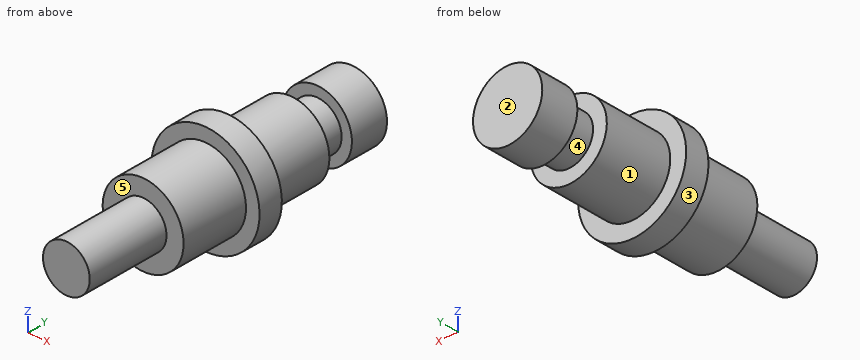
```python
from build123d import *

# Parameters (mm, degrees)
SKETCH1_R           = 4.77
BOSS_EXTRUDE1_DEPTH = 2.18
SKETCH2_R           = 3.575
BOSS_EXTRUDE2_DEPTH = 6.1
SKETCH3_R           = 2.065
BOSS_EXTRUDE3_DEPTH = 7.5
SKETCH4_R           = 3.365
BOSS_EXTRUDE4_DEPTH = 6.2
SKETCH5_R           = 2.15
BOSS_EXTRUDE5_DEPTH = 2.54
SKETCH6_R           = 3.06
BOSS_EXTRUDE6_DEPTH = 3.43


with BuildPart() as part:
    # Sketch1 → Boss-Extrude1 (new body)
    with BuildSketch(Plane(origin=(0, 0, 0), x_dir=(1, 0, 0), z_dir=(0, 1, 0))):
        with Locations(Location((0, 0, 0), (0, 0, 270))):
            Circle(SKETCH1_R)
    extrude(amount=BOSS_EXTRUDE1_DEPTH)

    # Sketch2 → Boss-Extrude2 (add)
    with BuildSketch(Plane.XZ):
        with Locations(Location((0, 0, 0), (0, 0, 90))):
            Circle(SKETCH2_R)
    extrude(amount=BOSS_EXTRUDE2_DEPTH)

    # Sketch3 → Boss-Extrude3 (add)
    with BuildSketch(Plane.XZ.offset(6.1)):
        with Locations(Location((0, 0, 0), (0, 0, 270))):
            Circle(SKETCH3_R)
    extrude(amount=BOSS_EXTRUDE3_DEPTH)

    # Sketch4 → Boss-Extrude4 (add)
    with BuildSketch(Plane(origin=(0, 2.18, 0), x_dir=(1, 0, 0), z_dir=(0, 1, 0))):
        with Locations(Location((0, 0, 0), (0, 0, 90))):
            Circle(SKETCH4_R)
    extrude(amount=BOSS_EXTRUDE4_DEPTH)

    # Sketch5 → Boss-Extrude5 (add)
    with BuildSketch(Plane(origin=(0, 8.38, 0), x_dir=(1, 0, 0), z_dir=(0, 1, 0))):
        with Locations(Location((0, 0, 0), (0, 0, 270))):
            Circle(SKETCH5_R)
    extrude(amount=BOSS_EXTRUDE5_DEPTH)

    # Sketch6 → Boss-Extrude6 (add)
    with BuildSketch(Plane(origin=(0, 10.92, 0), x_dir=(1, 0, 0), z_dir=(0, 1, 0))):
        with Locations(Location((0, 0, 0), (0, 0, 90))):
            Circle(SKETCH6_R)
    extrude(amount=BOSS_EXTRUDE6_DEPTH)


solid = part.part
```
Can you work these out from the model? Positions are in its coordinate system, mm. Face numbers are marked on the shaded views. A direction names the side the tool comes from. Give positions to 0.01 mm unless a question says otherwise; leave off trailing zeros. Write each loop counter-clockwise with the first axis right and the second up, starting at its lowest first coordinate (ties: lowest second). Pieces come first, ordered by that corner, then holes. Notation, with made-up numbers: (-0.75, -34.75) - (9.25, -34.75) arc R22 ccw to (9.25, -16.75) - close; hole circle Ø2 at (27, 2). An arc over 180 degrees is marked (long way). Write item = value, one per line. Start each with the question number.
1. Imagine slicing it at B-B (z = -2.75). Please give me the cut outline in (x, y), and give its area (3 significant figures).
2. Please list where these lines run through material, in increasing order: line 1 (Y direction, x = 0.25, z = 2.5); line 2 (Y direction, x = 2.5, z = -3.75); line 3 (Z direction, x = 2, y = -0.5).
3. Imagine slicing it at D-D (z = 0). Please give me the cut outline in (x, y) (3 decimals).
4. For pin 1 (1.5 mm diameter, centred on y = -2.5, z = 3, fed in from +X); pin 2 (3 mm diameter, centred on x = -1, y = -7, fed in from -Z) (3 decimals); pin 3 (4 mm diameter, centred on y = -4, z = 3, fed in from -X); pin 4 (1.5 mm diameter, centred on x = 3, y = -7, fed in from +Z), each with a flat end and sliding along its axis, tell me the tip position at first contact or that it passes through.
5. Imagine slicing it at A-A (x = 0). Please give me the cut outline in (y, z) (3 decimals).
6. On a 3-axis mill with a long thin cutter (end or side, diameter ignored), from which of +Z, -Z, +X, -X, +Y, -Y can I reach the whole of each face in a straight line? I mean the marked faces 1, 2, 3, 4 and 5. Say none if no direction works.
7. Imagine slicing it at C-C (x = -2.5). Please give me the cut outline in (y, z).
Worked answers:
q1.outline = (-3.9, 0) - (-2.28, 0) - (-2.28, -6.1) - (2.28, -6.1) - (2.28, 0) - (3.9, 0) - (3.9, 2.18) - (1.94, 2.18) - (1.94, 8.38) - (-1.94, 8.38) - (-1.94, 2.18) - (-3.9, 2.18) - close; (-1.34, 10.92) - (1.34, 10.92) - (1.34, 14.35) - (-1.34, 14.35) - close
q1.area = 78.1 mm2
q2.line_1 = -6.1 to 8.38, 10.92 to 14.35
q2.line_2 = 0 to 2.18
q2.line_3 = -2.96 to 2.96
q3.outline = (-4.77, 0) - (-3.575, 0) - (-3.575, -6.1) - (-2.065, -6.1) - (-2.065, -13.6) - (2.065, -13.6) - (2.065, -6.1) - (3.575, -6.1) - (3.575, 0) - (4.77, 0) - (4.77, 2.18) - (3.365, 2.18) - (3.365, 8.38) - (2.15, 8.38) - (2.15, 10.92) - (3.06, 10.92) - (3.06, 14.35) - (-3.06, 14.35) - (-3.06, 10.92) - (-2.15, 10.92) - (-2.15, 8.38) - (-3.365, 8.38) - (-3.365, 2.18) - (-4.77, 2.18) - close
q4.pin_1 = 2.78
q4.pin_2 = -3.575
q4.pin_3 = -3.43
q4.pin_4 = through
q5.outline = (-13.6, -2.065) - (-6.1, -2.065) - (-6.1, -3.575) - (0, -3.575) - (0, -4.77) - (2.18, -4.77) - (2.18, -3.365) - (8.38, -3.365) - (8.38, -2.15) - (10.92, -2.15) - (10.92, -3.06) - (14.35, -3.06) - (14.35, 3.06) - (10.92, 3.06) - (10.92, 2.15) - (8.38, 2.15) - (8.38, 3.365) - (2.18, 3.365) - (2.18, 4.77) - (0, 4.77) - (0, 3.575) - (-6.1, 3.575) - (-6.1, 2.065) - (-13.6, 2.065) - close
q6.face_1 = +Y
q6.face_2 = +Z, -Z, +X, -X, +Y
q6.face_3 = +Y, -Y
q6.face_4 = none
q6.face_5 = -Y
q7.outline = (-6.1, -2.56) - (0, -2.56) - (0, -4.06) - (2.18, -4.06) - (2.18, -2.25) - (8.38, -2.25) - (8.38, 2.25) - (2.18, 2.25) - (2.18, 4.06) - (0, 4.06) - (0, 2.56) - (-6.1, 2.56) - close; (10.92, -1.76) - (14.35, -1.76) - (14.35, 1.76) - (10.92, 1.76) - close
